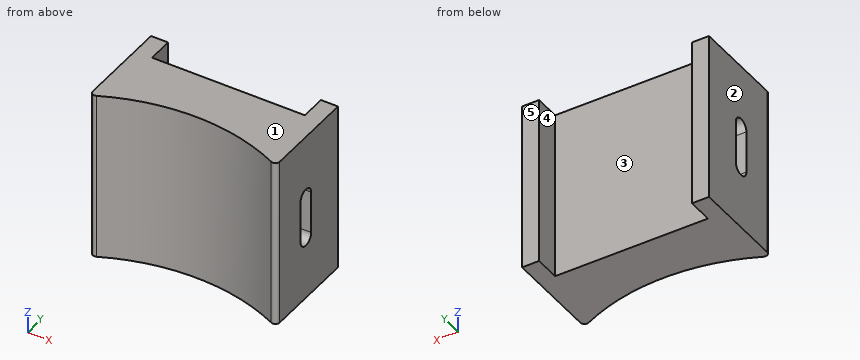
```python
from build123d import *

# Parameters (mm, degrees)
BOSS_EXTRUDE1_DEPTH = 20
CUT_EXTRUDE1_DEPTH  = 22.02


with BuildPart() as part:
    # Sketch1 → Boss-Extrude1 (new body)
    with BuildSketch(Plane.XY):
        with BuildLine():
            Line((-9, 3), (9, 3))
            Line((9, 3), (9, 6))
            Line((9, 6), (11.01, 6))
            Line((11.01, 6), (11.01, -4.883887969))
            ThreePointArc((11.01, -4.883887969), (10.776588402, -5.306889889), (10.294277504, -5.334957592))
            ThreePointArc((10.294277504, -5.334957592), (0, -3), (-10.294277504, -5.334957592))
            ThreePointArc((-10.294277504, -5.334957592), (-10.776588402, -5.306889889), (-11.01, -4.883887969))
            Line((-11.01, -4.883887969), (-11.01, 6))
            Line((-11.01, 6), (-9, 6))
            Line((-9, 6), (-9, 3))
        make_face()
    extrude(amount=BOSS_EXTRUDE1_DEPTH)

    # Sketch2 → Cut-Extrude1 (cut)
    with BuildSketch(Plane(origin=(11.01, 0, 0), x_dir=(0, 0, -1), z_dir=(1, 0, 0))):
        with BuildLine():
            Line((-12.5, 0.99), (-7.5, 0.99))
            ThreePointArc((-7.5, 0.99), (-6.51, 0), (-7.5, -0.99))
            Line((-7.5, -0.99), (-12.5, -0.99))
            ThreePointArc((-12.5, -0.99), (-13.49, 0), (-12.5, 0.99))
        make_face()
    extrude(amount=-CUT_EXTRUDE1_DEPTH, mode=Mode.SUBTRACT)


solid = part.part
```
The model under review builds one solid part; all positions refer to its coordinate system, in mm. Face numbers are marked on the shaded views. A direction names the side the tool comes from. Round coordinates to 2 decimals unless told otherwise and drop trailing zeros. Loops run counter-clockwise (first coordinate to the right, second up) from the corner with the lowest first, then second, coordinate; pieces in that order, holes last. Notation, with made-up numbers: (-2, 32.5) -> (17, 32.5) arc R29 cw to (17, 57.5) -> close; hole circle Ø6 at (-38, -23.5). An arc over 180 degrees is marked (long way). Answer as a JSON object with one key per item and string values. Group by question number.
1) We need section A-A on y = 4.25. Write out the cut boundary in (x, z), then the cut area to 3 significant figures.
2) We need section C-C on x = 4.25. Write out the cut boundary in (y, z).
3) For the marked faces 4 and 5, list the 3-axis set-ups (+Z, -Z, +X, -X, +Y, -Y) from which the entire face can be reached by the end or side of a thin tool; tool diameter is ignored.
4) Mouldability with a two-part tool opening along X and no side actions: class the marked faces 1, 2 and 3 as released by +X, released by -X, zero draft, split by the parting line, or undercut.
5) For pin 1 Ø5.5 at (x, z) = (-5, 10) entering from -Y; pin 2 Ø5.5 at (x, z) = (-0.5, 9.5) entering from +Y; pin 3 Ø1.5 at (x, z) = (-8.5, 9.5) entering from -Y, all flat-tipped, find the tip position at first contact; note any pin that passes through.
6) We need section D-D on z = 16.75. Write out the cut boundary in (x, y), then the cut area to 3 significant figures.
7) For line 1 (X direction, y = 4, z = 9.75); line 2 (Z direction, x = 0, y = 0); line 3 (Y direction, x = 5, z = 12.25), list the stretches that pass through material, from the lowest coordinate up. Write a range as [from, to].
8) We need section B-B on z = 8.5. Write out the cut boundary in (x, y), then the cut area to 3 significant figures.
Result set:
{
 "1": {"outline": "(-11.01, 0) -> (-9, 0) -> (-9, 20) -> (-11.01, 20) -> close; (9, 0) -> (11.01, 0) -> (11.01, 20) -> (9, 20) -> close", "area": "80.4 mm²"},
 "2": {"outline": "(-3.38, 0) -> (3, 0) -> (3, 20) -> (-3.38, 20) -> close; hole (-0.99, 7.5) arc R0.99 ccw to (0.99, 7.5) -> (0.99, 12.5) arc R0.99 ccw to (-0.99, 12.5) -> close"},
 "3": {"face 4": "+Z, -Z, +Y", "face 5": "+Z, -Z, +X, -X, +Y"},
 "4": {"face 1": "zero draft", "face 2": "released by -X", "face 3": "undercut"},
 "5": {"pin 1": "y = -4.29", "pin 2": "y = 3", "pin 3": "y = -4.87"},
 "6": {"outline": "(-11.01, -4.88) arc R0.5 ccw to (-10.29, -5.33) arc R23.86 cw to (10.29, -5.33) arc R0.5 ccw to (11.01, -4.88) -> (11.01, 6) -> (9, 6) -> (9, 3) -> (-9, 3) -> (-9, 6) -> (-11.01, 6) -> close", "area": "163 mm²"},
 "7": {"line 1": "[-11.01, -9], [9, 11.01]", "line 2": "[0, 6.51], [13.49, 20]", "line 3": "[-3.53, -0.99], [0.99, 3]"},
 "8": {"outline": "(-11.01, -4.88) arc R0.5 ccw to (-10.29, -5.33) arc R23.86 cw to (10.29, -5.33) arc R0.5 ccw to (11.01, -4.88) -> (11.01, -0.99) -> (-11.01, -0.99) -> close; (-11.01, 0.99) -> (11.01, 0.99) -> (11.01, 6) -> (9, 6) -> (9, 3) -> (-9, 3) -> (-9, 6) -> (-11.01, 6) -> close", "area": "120 mm²"}
}
